Could you check a few things on this model? Use its own coordinates, in mm. A direction names the side the tool comes from. Coordinates: 2 decimals unless noted, no trailing zeros. Write each loop counter-clockwise with the first axis right and the second up, starting at its lowest first coordinate (ties: lowest second). Pieces come first, ordered by that corner, then holes. Notation, with made-up numbers: (85, -24.75) - (125, -24.75) arc R19 ccw to (125, -20.75) - close; hole circle Ø9 at (12, 50). An arc over 180 degrees is marked (long way). Write item = value, one per line. Start each with the question number.
```python
from build123d import *

# Parameters (mm, degrees)
SKETCH1_R           = 30
BOSS_EXTRUDE1_DEPTH = 5
SKETCH2_R           = 2
BOSS_EXTRUDE2_DEPTH = 13
BOSS_EXTRUDE3_DEPTH = 15


with BuildPart() as part:
    # Sketch1 → Boss-Extrude1 (new body)
    with BuildSketch(Plane(origin=(0, 0, 0), x_dir=(1, 0, 0), z_dir=(0, 1, 0))):
        with Locations(Location((0, 0, 0), (0, 0, 270))):
            Circle(SKETCH1_R)
    extrude(amount=BOSS_EXTRUDE1_DEPTH)

    # Sketch2 → Boss-Extrude2 (add)
    with BuildSketch(Plane(origin=(0, 5, 0), x_dir=(1, 0, 0), z_dir=(0, 1, 0))):
        with Locations(Location((0, 25, 0), (0, 0, 90))):
            Circle(SKETCH2_R)
        with Locations(Location((21.650635095, 12.5, 0), (0, 0, 90))):
            Circle(SKETCH2_R)
        with Locations(Location((21.650635095, -12.5, 0), (0, 0, 90))):
            Circle(SKETCH2_R)
        with Locations(Location((0, -25, 0), (0, 0, 90))):
            Circle(SKETCH2_R)
        with Locations(Location((-21.650635095, -12.5, 0), (0, 0, 90))):
            Circle(SKETCH2_R)
        with Locations(Location((-21.650635095, 12.5, 0), (0, 0, 90))):
            Circle(SKETCH2_R)
    extrude(amount=BOSS_EXTRUDE2_DEPTH)

    # Sketch3 → Boss-Extrude3 (add)
    with BuildSketch(Plane.XZ):
        with BuildLine():
            Line((-10, 20), (10, 20))
            Line((10, 20), (10, 11.180339887))
            ThreePointArc((10, 11.180339887), (0, -15), (-10, 11.180339887))
            Line((-10, 11.180339887), (-10, 20))
        make_face()
    extrude(amount=BOSS_EXTRUDE3_DEPTH)


solid = part.part
```
1) Suppose I cut it at C-C on x = 8. Please give me the cut outline in (y, z).
2) Which directions (+Z, -Z, +X, -X, +Y, -Y) give clear straight access to the entire face, cutting with the end or side of a thin tool? Please do faces 1 (the cylindrical face through (23.603, 11.409, 12.934)), 2 (the flat face through (10, -7, 16)), 3 (the cylindrical face through (0.51, -7.4, -14.99)).
3) If I drill on probe 1 along Y at (x, z) = (-19.5, 22); probe 2 along Y at (x, z) = (8.5, 4); probe 3 along X at (y, z) = (-9.5, -10), over which ranges is the centre line in solid material (lowest first)? Write a range as [from, to].
4) Suppose I cut it at A-A on z = 0. Please give me the cut outline in (x, y), plus the area to 3 significant figures.
5) Suppose I cut it at D-D on x = 0. Please give me the cut outline in (y, z).
6) Suppose I cut it at B-B on y = 13. Please give me the cut outline in (x, z), plus the area to 3 significant figures.
7) Thinking about a two-plate mould opening in Z: for faces 4 (the cylindrical face through (1.32, 2.46, -29.97)), 5 (the flat face through (-6, 0, -14)), 6 (the flat face through (0, -7, 20)), 7 (the cylindrical face through (-19.698, 11.409, 12.934)), which applies, +Z half, -Z half, draft (parallel to the pull), parting line (faces both ways), or undercut?
8) For P1, Ø5, axis at x = -22, z = -23.5, coming from the +Y side; P2, Ø5, axis at x = -11.5, y = 0.5, coming from the -Z side; P3, Ø10, axis at y = -8.5, z = 15, coming from the -X side; P4, Ø1.5, axis at y = 13, z = -22, coming from the -X side, each with a flat end and sliding along its axis, tell me the tip position at first contact or that it passes through.
Reply:
q1.outline = (-15, -12.69) - (0, -12.69) - (0, -28.91) - (5, -28.91) - (5, 28.91) - (0, 28.91) - (0, 20) - (-15, 20) - close
q2.face_1 = +Y
q2.face_2 = +Z, +X, -Y
q2.face_3 = -Y
q3.probe_1 = [0, 5]
q3.probe_2 = [-15, 5]
q3.probe_3 = [-11.18, 11.18]
q4.outline = (-30, 0) - (-15, 0) - (-15, -15) - (15, -15) - (15, 0) - (30, 0) - (30, 5) - (-30, 5) - close
q4.area = 750 mm^2
q5.outline = (-15, -15) - (0, -15) - (0, -30) - (5, -30) - (5, -27) - (18, -27) - (18, -23) - (5, -23) - (5, 23) - (18, 23) - (18, 27) - (5, 27) - (5, 30) - (0, 30) - (0, 20) - (-15, 20) - close
q6.outline = circle Ø4 at (-21.65, -12.5); circle Ø4 at (-21.65, 12.5); circle Ø4 at (0, -25); circle Ø4 at (0, 25); circle Ø4 at (21.65, -12.5); circle Ø4 at (21.65, 12.5)
q6.area = 75.4 mm^2
q7.face_4 = parting line
q7.face_5 = draft
q7.face_6 = +Z half
q7.face_7 = undercut
q8.P1 = 5
q8.P2 = -28.62
q8.P3 = -11.18
q8.P4 = through
